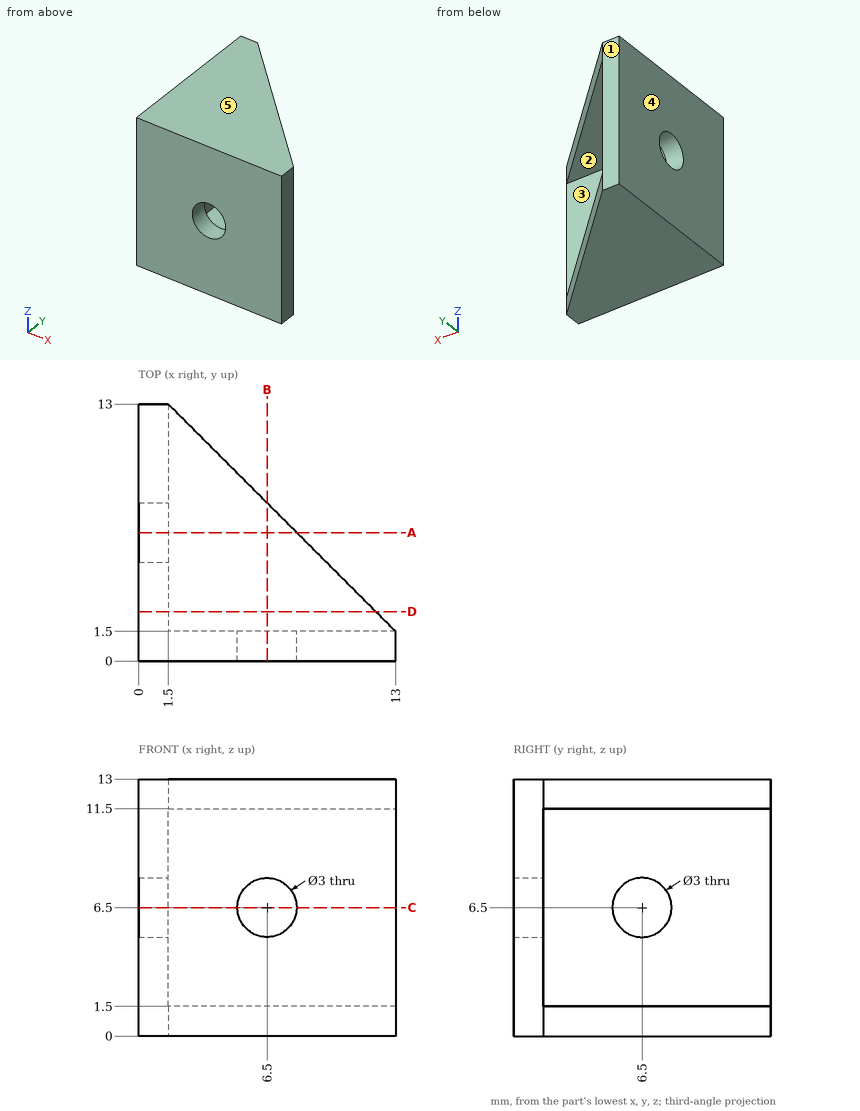
Study the drawing (mm; zero at the part's minimum x, y, z) and answer. A direction names the side the tool comes from. Give positions to 0.01 mm unless a question says otherwise; leave off trailing zeros. Order: outer loops, then holes, each group sorted by start corner. A loop starts at its lowest first (then second) coordinate and runs counter-clockwise, first axis right, second up.
1) For the marked faces 1 and 2, determine the directions among +Z, -Z, +X, -X, +Y, -Y from which every point of the face is accessible in a straight line to the end or side of a thin tool.
Reported:
face 1: +Z, -Z, +X, -X, +Y
face 2: +X, +Y
2) Find section D-D on y = 2.5. Write down the section's boundary in (x, z).
Reported:
outline: (0, 0) - (12, 0) - (12, 1.5) - (1.5, 1.5) - (1.5, 11.5) - (12, 11.5) - (12, 13) - (0, 13) - close
3) Find section C-C on z = 6.5. Write down the section's boundary in (x, y), then the cut area to 4 significant figures.
Reported:
outline: (0, 0) - (5, 0) - (5, 1.5) - (1.5, 1.5) - (1.5, 5) - (0, 5) - close; (0, 8) - (1.5, 8) - (1.5, 13) - (0, 13) - close; (8, 0) - (13, 0) - (13, 1.5) - (8, 1.5) - close
area: 27.75 mm2
4) Consider line 1 along X through (y, z) = (0.3, 6.5); line 2 along Z through (x, y) = (4.25, 7). Determine where each line is inside the solid, lowest interval first.
Reported:
line 1: x = 0 to 5, 8 to 13
line 2: z = 0 to 1.5, 11.5 to 13
5) Determine the mould class of the marked faces 3, 4 and 5 for opening direction Z: pulls with the +Z half, pulls with the -Z half, needs draft (parallel to the pull), parting line crosses it, or undercut.
Reported:
face 3: undercut
face 4: needs draft
face 5: pulls with the +Z half
6) Given P1, Ø5, axis at y = 9.5, z = 5.5, coming from the +X side; P2, Ø3, axis at x = 5.5, z = 8, coming from the +Y side; P3, Ø1.8, axis at y = 6.5, z = 6.5, coming from the +X side, each flat-ended and moving along its own axis, determine where each tip first touches the part or whether it passes through.
Reported:
P1: stops at x = 1.5
P2: stops at y = 1.5
P3: passes through
7) Find section A-A on y = 6.5. Write down the section's boundary in (x, z), then the cut area to 3 significant figures.
Reported:
outline: (0, 0) - (8, 0) - (8, 1.5) - (1.5, 1.5) - (1.5, 5) - (0, 5) - close; (0, 8) - (1.5, 8) - (1.5, 11.5) - (8, 11.5) - (8, 13) - (0, 13) - close
area: 34.5 mm2
